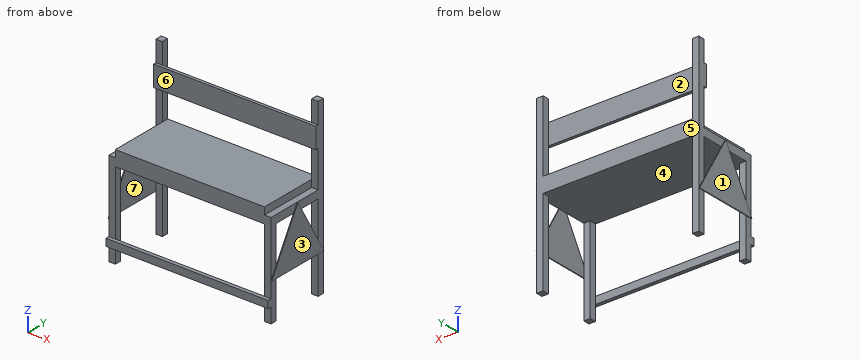
```python
from build123d import *

# Parameters (mm, degrees)
F0_W      = 1130
F0_H      = 450
F1_DEPTH  = 55
F2_W      = 45
F2_H      = 45
F3_DEPTH  = 600
F4_W      = 45
F4_H      = 45
F5_DEPTH  = 600
F6_W      = 45
F6_H      = 45
F7_DEPTH  = 600
F8_W      = 45
F8_H      = 45
F9_DEPTH  = 600
F10_W     = 45
F10_H     = 45
F11_DEPTH = 545
F12_W     = 45
F12_H     = 45
F13_DEPTH = 545
F14_W     = 1130
F14_H     = 145
F15_DEPTH = 20
F16_W     = 1130
F16_H     = 50
F17_DEPTH = 25
F18_W     = 1040
F18_H     = 450
F19_DEPTH = 50
F21_DEPTH = 5
F23_DEPTH = 5


with BuildPart() as f1:
    # F0 (on Top) → F1 (new body)
    with BuildSketch(Plane.XY):
        with Locations((-10.878954, -127.968649)):
            Rectangle(F0_W, F0_H)
    extrude(amount=F1_DEPTH)

    # F2 (on face) → F3 (join)
    with BuildSketch(Plane(origin=(0, 0, 0), x_dir=(1, 0, 0), z_dir=(0, 0, -1))):
        with Locations((531.621046, -74.531351)):
            Rectangle(F2_W, F2_H)
    extrude(amount=F3_DEPTH)

    # F4 (on face) → F5 (join)
    with BuildSketch(Plane(origin=(0, 0, 0), x_dir=(1, 0, 0), z_dir=(0, 0, -1))):
        with Locations((-553.378954, -74.531351)):
            Rectangle(F4_W, F4_H)
    extrude(amount=F5_DEPTH)

    # F6 (on face) → F7 (join)
    with BuildSketch(Plane(origin=(0, 0, 0), x_dir=(1, 0, 0), z_dir=(0, 0, -1))):
        with Locations((531.621046, 330.468649)):
            Rectangle(F6_W, F6_H)
    extrude(amount=F7_DEPTH)

    # F8 (on face) → F9 (join)
    with BuildSketch(Plane(origin=(0, 0, 0), x_dir=(1, 0, 0), z_dir=(0, 0, -1))):
        with Locations((-553.378954, 330.468649)):
            Rectangle(F8_W, F8_H)
    extrude(amount=F9_DEPTH)

    # F10 (on face) → F11 (join)
    with BuildSketch(Plane.XY.offset(55)):
        with Locations((531.621046, 74.531351)):
            Rectangle(F10_W, F10_H)
    extrude(amount=F11_DEPTH)

    # F12 (on face) → F13 (join)
    with BuildSketch(Plane.XY.offset(55)):
        with Locations((-553.378954, 74.531351)):
            Rectangle(F12_W, F12_H)
    extrude(amount=F13_DEPTH)

    # F14 (on face) → F15 (join)
    with BuildSketch(Plane.XZ.offset(-52.031351)):
        with Locations((-10.878954, 382.5)):
            Rectangle(F14_W, F14_H)
    extrude(amount=F15_DEPTH)

    # F16 (on face) → F17 (join)
    with BuildSketch(Plane.XZ.offset(352.968649)):
        with Locations((-10.878954, -470.051563)):
            Rectangle(F16_W, F16_H)
    extrude(amount=F17_DEPTH)

    # F18 (on face) → F19 (join)
    with BuildSketch(Plane.XY.offset(55)):
        with Locations((-10.878954, -127.968649)):
            Rectangle(F18_W, F18_H)
    extrude(amount=F19_DEPTH)

    # F20 (on face) → F21 (join)
    with BuildSketch(Plane.YZ.offset(554.121046)):
        Polygon((-127.968649, 55), (-352.968649, -335), (97.031351, -335), align=None)
    extrude(amount=F21_DEPTH)

    # F22 (on face) → F23 (join)
    with BuildSketch(Plane(origin=(-575.878954, 0, 0), x_dir=(0, -1, 0), z_dir=(-1, 0, 0))):
        Polygon((-97.031351, -335), (352.968649, -335), (127.968649, 55), align=None)
    extrude(amount=F23_DEPTH)


solid = f1.part
```
The model under review builds one solid part; all positions refer to its coordinate system, in mm. Face numbers are marked on the shaded views. A direction names the side the tool comes from. Coordinates: 2 decimals unless noted, no trailing zeros. Write each loop counter-clockwise with the first axis right and the second up, starting at its lowest first coordinate (ties: lowest second). Pieces come first, ordered by that corner, then holes. Notation, with made-up numbers: (30.5, -13) -> (70.5, -13) arc R28 cw to (70.5, 6) -> close; hole circle Ø5 at (22, 21.25). An arc over 180 degrees is marked (long way). One line per item, written item: value. Start each with the question number.
Q1. Add section B-B, the plane z = 86.5. Give the boundary of the cut face in (x, y), then the cut area to 3 significant figures.
Q2. Add section D-D, the plane z = -374. Give the boundary of the cut face in (x, y), then the cut area to 3 significant figures.
Q3. Add section C-C, the plane y = -221.5. Give the boundary of the cut face in (x, z), then the cut area to 3 significant figures.
Q4. Add section A-A, the plane x = -221.5. Give the boundary of the cut face in (y, z).
Q5. Clearance check with flat-ended pins moving along their axes: P1, Ø13.5, axis at y = -338, z = -181, coming from the -X side; P2, Ø4, axis at x = 556.5, y = -139.5, coming from the -Z side; P3, Ø3, axis at x = 201, y = -168, coming from the +Z side. State where each tip first meets the part, or that it passes through.
Q6. To check wall thickness, follow probe 1 along X at (y, z) = (-80.5, -81); probe 2 along X at (y, z) = (57, 514); probe 3 along Y at (x, z) = (98, 400). State the ranges of each line that lie inside material, in increasing order.
Q7. The part is to be moulded in two halves that separate along X. For the marked faces 1, 2, 3 and 4, say which applies: +X half, -X half, draft (parallel to the pull), parting line (faces both ways), or undercut.
Q8. For the marked faces 5, 6 and 7, list the 3-axis set-ups (+Z, -Z, +X, -X, +Y, -Y) from which the entire face can be reached by the end or side of a thin tool; tool diameter is ignored.
Response:
1. outline: (-575.88, 52.03) -> (-530.88, 52.03) -> (-530.88, -352.97) -> (509.12, -352.97) -> (509.12, 52.03) -> (554.12, 52.03) -> (554.12, 97.03) -> (-575.88, 97.03) -> close
1. area: 472,000 mm²
2. outline: (-575.88, -352.97) -> (-530.88, -352.97) -> (-530.88, -307.97) -> (-575.88, -307.97) -> close; (-575.88, 52.03) -> (-530.88, 52.03) -> (-530.88, 97.03) -> (-575.88, 97.03) -> close; (509.12, -352.97) -> (554.12, -352.97) -> (554.12, -307.97) -> (509.12, -307.97) -> close; (509.12, 52.03) -> (554.12, 52.03) -> (554.12, 97.03) -> (509.12, 97.03) -> close
2. area: 8,100 mm²
3. outline: (-580.88, -335) -> (-575.88, -335) -> (-575.88, -107.12) -> (-580.88, -107.12) -> close; (-575.88, 0) -> (554.12, 0) -> (554.12, 55) -> (509.12, 55) -> (509.12, 105) -> (-530.88, 105) -> (-530.88, 55) -> (-575.88, 55) -> close; (554.12, -335) -> (559.12, -335) -> (559.12, -107.12) -> (554.12, -107.12) -> close
3. area: 116,000 mm²
4. outline: (-377.97, -495.05) -> (-352.97, -495.05) -> (-352.97, -445.05) -> (-377.97, -445.05) -> close; (-352.97, 0) -> (97.03, 0) -> (97.03, 105) -> (-352.97, 105) -> close; (32.03, 310) -> (52.03, 310) -> (52.03, 455) -> (32.03, 455) -> close
5. P1: x = -575.88
5. P2: z = -335
5. P3: z = 105
6. probe 1: -580.88 to -575.88, 554.12 to 559.12
6. probe 2: -575.88 to -530.88, 509.12 to 554.12
6. probe 3: 32.03 to 52.03
7. face 1: -X half
7. face 2: undercut
7. face 3: +X half
7. face 4: undercut
8. face 5: +Z, -Z, +X, -X, +Y
8. face 6: +Z, +X, -X, -Y
8. face 7: -Z
